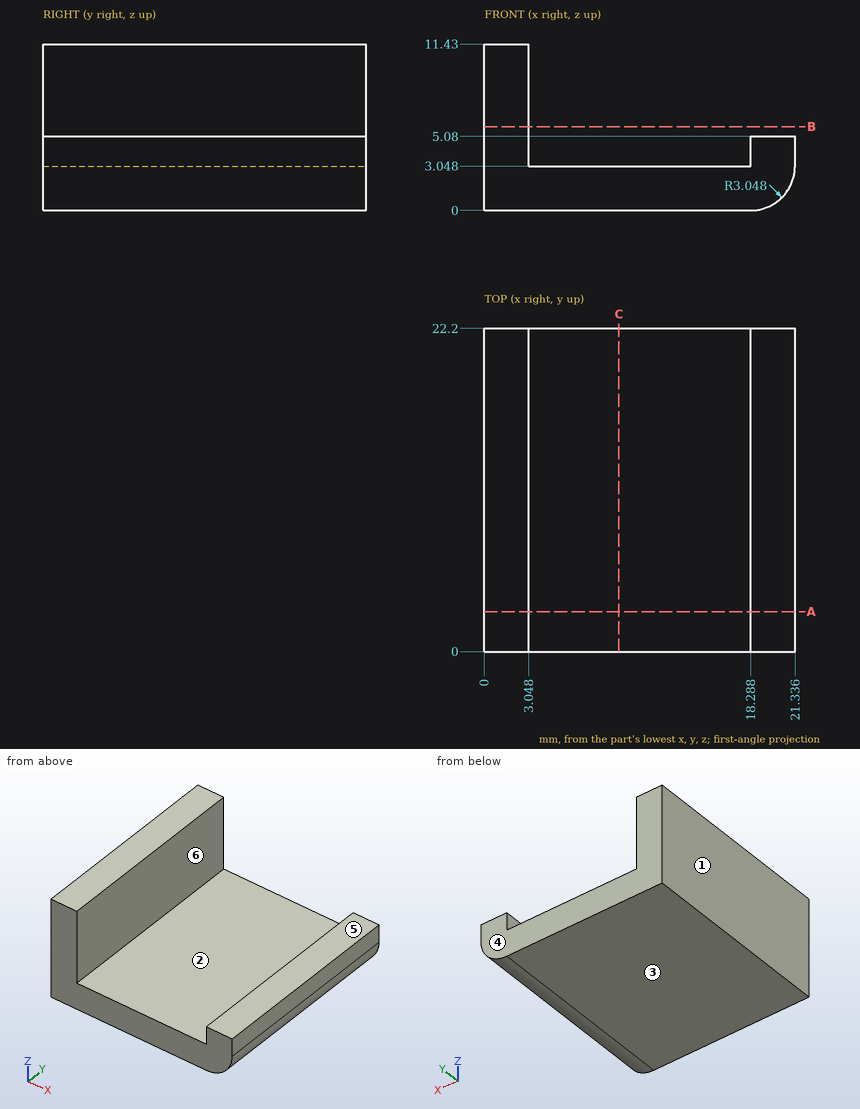
Source: three-view drawing plus pictorial views. Frame: mm from the lowest corner of the part. A direction names the side the tool comes from. Coordinates: 2 decimals unless noted, no trailing zeros. Loops run counter-clockwise (first coordinate to the right, second up) from the corner with the lowest first, then second, coordinate; pieces in that order, holes last. Notation, with made-up numbers: (75.5, 17.25) -> (109.5, 17.25) arc R15 cw to (109.5, 31.25) -> close; hole circle Ø1 at (-40, 52.25). An arc over 180 degrees is marked (long way). Answer in a Markdown table with one row per item. Add a question column.
Q1. Pull-direction query (X, two-part tool) for the marked faces 1, 2 and 3; classes: pulls with the +X half, pulls with the -X half, needs draft (parallel to the pull), parting line crosses it, or undercut.
Q2. Ray query, line 1 along X through (y, z) = (15.5, 5); line 2 along X through (y, z) = (18, 6.5). Return the intervals inside material, ascending.
Q3. Section B-B on z = 5.75. Return the cut outline in (x, y).
Q4. Reachability of the marked faces 4, 5 and 6 from +Z, -Z, +X, -X, +Y, -Y: full face, straight path, thin tool, end or side. Return the list, or none.
Q5. Contact query for flat-ended pins moving along their axis: pin 1 Ø4 at (x, z) = (2.5, 5) entering from -Y; pin 2 Ø2.5 at (y, z) = (13, 9) entering from +X; pin 3 Ø5 at (x, y) = (6.5, 3.5) entering from +Z; pin 4 Ø0.9 at (x, y) = (19.5, 7.5) entering from +Z. Output: stop coordinate, or through.
Q6. Section A-A on y = 2.75. Return the cut outline in (x, z).
Q7. Section C-C on x = 9.25. Return the cut outline in (y, z).
Computed values:
| question | item | result |
|---|---|---|
| 1 | face 1 | pulls with the -X half |
| 1 | face 2 | undercut |
| 1 | face 3 | needs draft |
| 2 | line 1 | x = 0 to 3.05, 18.29 to 21.34 |
| 2 | line 2 | x = 0 to 3.05 |
| 3 | outline | (0, 0) -> (3.05, 0) -> (3.05, 22.2) -> (0, 22.2) -> close |
| 4 | face 4 | +Z, -Z, +X, -X, +Y |
| 4 | face 5 | +Z, +X, +Y, -Y |
| 4 | face 6 | +Z, +Y, -Y |
| 5 | pin 1 | stops at y = 0 |
| 5 | pin 2 | stops at x = 3.05 |
| 5 | pin 3 | stops at z = 3.05 |
| 5 | pin 4 | stops at z = 5.08 |
| 6 | outline | (0, 0) -> (18.29, 0) arc R3.05 ccw to (21.34, 3.05) -> (21.34, 5.08) -> (18.29, 5.08) -> (18.29, 3.05) -> (3.05, 3.05) -> (3.05, 11.43) -> (0, 11.43) -> close |
| 7 | outline | (0, 0) -> (22.2, 0) -> (22.2, 3.05) -> (0, 3.05) -> close |
